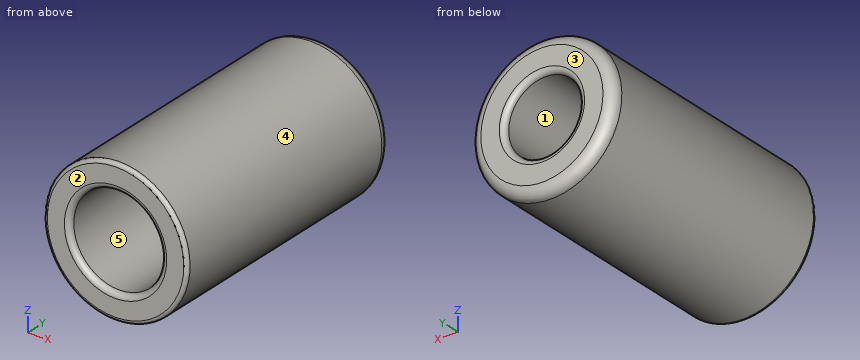
```python
from build123d import *

# Parameters (mm, degrees)
SKETCH1_R           = 20
BOSS_EXTRUDE1_DEPTH = 35
SKETCH2_R           = 12.75
CUT_EXTRUDE1_DEPTH  = 35
SKETCH3_R           = 20
BOSS_EXTRUDE2_DEPTH = 5
SKETCH4_R           = 12.75
CUT_EXTRUDE2_DEPTH  = 10
CUT_EXTRUDE2_DRAFT  = -45
SKETCH5_R           = 20
BOSS_EXTRUDE3_DEPTH = 35
SKETCH6_R           = 10.375
CUT_EXTRUDE3_DEPTH  = 33
FILLET1_R           = 1.5
FILLET2_R           = 1.5
FILLET3_R           = 3
FILLET4_R           = 1


with BuildPart() as part:
    # Sketch1 → Boss-Extrude1 (new body)
    with BuildSketch(Plane(origin=(0, 0, 0), x_dir=(1, 0, 0), z_dir=(0, 1, 0))):
        with Locations(Location((0, 0, 0), (0, 0, 270))):
            Circle(SKETCH1_R)
    extrude(amount=BOSS_EXTRUDE1_DEPTH)

    # Sketch2 → Cut-Extrude1 (cut)
    with BuildSketch(Plane.XZ):
        with Locations(Location((0, 0, 0), (0, 0, 270))):
            Circle(SKETCH2_R)
    extrude(amount=-CUT_EXTRUDE1_DEPTH, mode=Mode.SUBTRACT)

    # Sketch3 → Boss-Extrude2 (add)
    with BuildSketch(Plane(origin=(0, 35, 0), x_dir=(1, 0, 0), z_dir=(0, 1, 0))):
        with Locations(Location((0, 0, 0), (0, 0, 270))):
            Circle(SKETCH3_R)
    extrude(amount=BOSS_EXTRUDE2_DEPTH)


with BuildPart() as cut_extrude2_tool:
    # Sketch4 → Cut-Extrude2 (with draft: the straight prism first)
    with BuildSketch(Plane.XZ.offset(-35)):
        with Locations(Location((0, 0, 0), (0, 0, 270))):
            Circle(SKETCH4_R)
    extrude(amount=-CUT_EXTRUDE2_DEPTH)
    # Cut-Extrude2: the draft: its side faces are tilted about the plane it starts from
    cut_extrude2_sides = [cut_extrude2_tool.faces().sort_by_distance(p)[0] for p in [
        (0, 40, 12.75),
    ]]
    draft(cut_extrude2_sides, Plane.XZ.offset(-35), CUT_EXTRUDE2_DRAFT)


with BuildPart() as part_1:
    add(part.part)

    # Cut-Extrude2: cut by cut_extrude2_tool
    add(cut_extrude2_tool.part, mode=Mode.SUBTRACT)

    # Sketch5 → Boss-Extrude3 (add)
    with BuildSketch(Plane(origin=(0, 40, 0), x_dir=(1, 0, 0), z_dir=(0, 1, 0))):
        with Locations(Location((0, 0, 0), (0, 0, 270))):
            Circle(SKETCH5_R)
    extrude(amount=BOSS_EXTRUDE3_DEPTH)

    # Sketch6 → Cut-Extrude3 (cut)
    with BuildSketch(Plane(origin=(0, 75, 0), x_dir=(1, 0, 0), z_dir=(0, 1, 0))):
        with Locations(Location((0, 0, 0), (0, 0, 270))):
            Circle(SKETCH6_R)
    extrude(amount=-CUT_EXTRUDE3_DEPTH, mode=Mode.SUBTRACT)

    # Fillet1
    fillet1_edges = [part_1.edges().sort_by_distance(p)[0] for p in [
        (0, 0, 12.75),
    ]]
    fillet(fillet1_edges, radius=FILLET1_R)

    # Fillet2
    fillet2_edges = [part_1.edges().sort_by_distance(p)[0] for p in [
        (0, 75, -10.375),
    ]]
    fillet(fillet2_edges, radius=FILLET2_R)

    # Fillet3
    fillet3_edges = [part_1.edges().sort_by_distance(p)[0] for p in [
        (0, 75, -20),
    ]]
    fillet(fillet3_edges, radius=FILLET3_R)

    # Fillet4
    fillet4_edges = [part_1.edges().sort_by_distance(p)[0] for p in [
        (0, 0, -20),
    ]]
    fillet(fillet4_edges, radius=FILLET4_R)


solid = part_1.part
```
Can you work these out from the model? Positions are in its coordinate system, mm. Face numbers are marked on the shaded views. A direction names the side the tool comes from. Coordinates: 2 decimals unless noted, no trailing zeros. Loops run counter-clockwise (first coordinate to the right, second up) from the corner with the lowest first, then second, coordinate; pieces in that order, holes last.
1) Which directions (+Z, -Z, +X, -X, +Y, -Y) give clear straight access to the entire face, cutting with the end or side of a thin tool? Please do the marked faces 1 and 2.
2) For pin 1 (1.5 mm diameter, centred on y = 52, z = -12.5, fed in from -X); pin 2 (12 mm diameter, centred on y = 10, z = -15, fed in from +X); pin 3 (6 mm diameter, centred on x = -0.5, z = -4.5, fed in from +Y), each with a flat end and sliding along its axis, tell me the tip position at first contact or that it passes through.
3) Imagine slicing it at B-B on z = 0. List the corners of the cut face in (x, y) for me (3 decimals), plus the area to 3 significant figures.
4) Imagine slicing it at D-D on y = 10. List the corners of the cut face in (x, z) for me.
5) I need wall thicknesses on probe 1 along X at (y, z) = (12.5, 0); probe 2 along X at (y, z) = (52, 0) (3 decimals); probe 3 along Y at (x, z) = (-13.5, 4). Which ranges of each line are inside material? Lowest first, please.
6) Thinking about a two-plate mould opening in X: for the marked faces 3, 4 and 5, which applies, pulls with the +X half, pulls with the -X half, needs draft (parallel to the pull), parting line crosses it, or undercut?
7) Imagine slicing it at A-A on x = 0. List the corners of the cut face in (y, z) for me (3 decimals), plus the area to 3 significant figures.
8) Imagine slicing it at C-C on y = 64. List the corners of the cut face in (x, z) for me (3 decimals), plus the area to 3 significant figures.
Completed:
1. face 1: +Y
1. face 2: +Z, -Z, +X, -X, -Y
2. pin 1: stops at x = -16.18
2. pin 2: stops at x = 17.86
2. pin 3: stops at y = 42
3. outline: (-20, 1) arc R1 ccw to (-19, 0) - (-14.25, 0) arc R1.5 ccw to (-12.75, 1.5) - (-12.75, 35) - (-7.75, 40) - (7.75, 40) - (12.75, 35) - (12.75, 1.5) arc R1.5 ccw to (14.25, 0) - (19, 0) arc R1 ccw to (20, 1) - (20, 72) arc R3 ccw to (17, 75) - (11.875, 75) arc R1.5 ccw to (10.375, 73.5) - (10.375, 42) - (-10.375, 42) - (-10.375, 73.5) arc R1.5 ccw to (-11.875, 75) - (-17, 75) arc R3 ccw to (-20, 72) - close
3. area: 1,310 mm2
4. outline: circle Ø40 at (0, 0); hole circle Ø25.5 at (0, 0)
5. probe 1: x = -20 to -12.75, 12.75 to 20
5. probe 2: x = -20 to -10.375, 10.375 to 20
5. probe 3: y = 0.01 to 75
6. face 3: needs draft
6. face 4: parting line crosses it
6. face 5: undercut
7. outline: (0, -19) arc R1 ccw to (1, -20) - (72, -20) arc R3 ccw to (75, -17) - (75, -11.875) arc R1.5 ccw to (73.5, -10.375) - (42, -10.375) - (42, 10.375) - (73.5, 10.375) arc R1.5 ccw to (75, 11.875) - (75, 17) arc R3 ccw to (72, 20) - (1, 20) arc R1 ccw to (0, 19) - (0, 14.25) arc R1.5 ccw to (1.5, 12.75) - (35, 12.75) - (40, 7.75) - (40, -7.75) - (35, -12.75) - (1.5, -12.75) arc R1.5 ccw to (0, -14.25) - close
7. area: 1,310 mm2
8. outline: circle Ø40 at (0, 0); hole circle Ø20.75 at (0, 0)
8. area: 918 mm2
